Input: part model. Units: mm. Frame: model coordinates. A direction names the side the tool comes from. Round coordinates to 2 decimals unless told otherwise and drop trailing zeros. Write each loop counter-clockwise with the first axis right and the second up, starting at its lowest first coordinate (ties: lowest second). Pieces come first, ordered by that corner, then holes. Notation, with made-up numbers: (-2, 17) -> (40, 17) arc R3 cw to (40, 21) -> close; hole circle Ø3 at (-39.5, -8). An arc over 180 degrees is marked (long way). Write item = value, one per line. Start each with the question number.
```python
from build123d import *

# Parameters (mm, degrees)
F1_DEPTH = 5


with BuildPart() as f1:
    # F0 (on Front) → F1 (new body)
    with BuildSketch(Plane.XZ):
        Polygon((25, 41.161765), (25, 58.161765), (-25, 58.161765), (-25, 41.161765), (-30, 41.161765), (-30, 24.161765), (-25, 24.161765), (-25, 7.161765), (-30, 7.161765), (-30, -9.838235), (-25, -9.838235), (-25, -26.838235), (-10, -26.838235), (-10, -31.838235), (-10, -36.838235), (10, -36.838235), (10, -31.838235), (10, -26.838235), (25, -26.838235), (25, -9.838235), (30, -9.838235), (30, 7.161765), (25, 7.161765), (25, 24.161765), (30, 24.161765), (30, 41.161765), align=None)
    extrude(amount=F1_DEPTH)


solid = f1.part
```
1. Line query: line 1 along Z through (x, y) = (27.5, -1.9); line 2 along Z through (x, y) = (-14.5, -3.7); line 3 along X through (y, z) = (-4.6, 47). Output: solid intervals per line, ascending.
2. Section B-B (x = 22). Output: boundary loops of the cut face in (y, z).
3. Section A-A (y = -3.5). Output: boundary loops of the cut face in (x, z).
4. Section C-C (z = 9). Output: boundary loops of the cut face in (x, y).
5. Reachability of faces 4 (the flat face through (-25, -2, 50)), 5 (the flat face through (25, -2, 16)), 6 (the flat face through (-28, -2, 24.162)) from +Z, -Z, +X, -X, +Y, -Y: full face, straight path, thin tool, end or side. Return the list, or none.
6. Mould query, pull axis Z, two halves, no side actions, for faces 1 (the flat face through (-27, -2, 41.162)), 2 (the flat face through (30, -2, 33)), 3 (the flat face through (-25, -2, 16)). Classes: pulls with the +Z half, pulls with the -Z half, needs draft (parallel to the pull), parting line crosses it, or undercut.
7. Pin query (flat end, axial travel): P1, Ø2.5, axis at x = 27, y = -2, coming from the +Z side; P2, Ø1.5, axis at x = -28.5, y = -1.5, coming from the -Z side; P3, Ø1.5, axis at y = -3, z = -18, coming from the -X side. Return the tip coordinate at first contact, or that it passes through.
Check sheet entries:
q1.line_1 = -9.84 to 7.16, 24.16 to 41.16
q1.line_2 = -26.84 to 58.16
q1.line_3 = -25 to 25
q2.outline = (-5, -26.84) -> (0, -26.84) -> (0, 58.16) -> (-5, 58.16) -> close
q3.outline = (-30, -9.84) -> (-25, -9.84) -> (-25, -26.84) -> (-10, -26.84) -> (-10, -36.84) -> (10, -36.84) -> (10, -26.84) -> (25, -26.84) -> (25, -9.84) -> (30, -9.84) -> (30, 7.16) -> (25, 7.16) -> (25, 24.16) -> (30, 24.16) -> (30, 41.16) -> (25, 41.16) -> (25, 58.16) -> (-25, 58.16) -> (-25, 41.16) -> (-30, 41.16) -> (-30, 24.16) -> (-25, 24.16) -> (-25, 7.16) -> (-30, 7.16) -> close
q4.outline = (-25, -5) -> (25, -5) -> (25, 0) -> (-25, 0) -> close
q5.face_4 = +Z, -X, +Y, -Y
q5.face_5 = +X, +Y, -Y
q5.face_6 = -X, +Y, -Y
q6.face_1 = pulls with the +Z half
q6.face_2 = needs draft
q6.face_3 = undercut
q7.P1 = 41.16
q7.P2 = -9.84
q7.P3 = -25
